Verification items for this drawing (mm, ordinates from the low corner). A direction names the side the tool comes from. Coordinates: 2 decimals unless noted, no trailing zeros. Order: outer loops, then holes, each group sorted by start corner. A loop starts at its lowest first (then second) coordinate and runs counter-clockwise, first axis right, second up. Notation, with made-up numbers: M 19.5,-7.5 L 78.5,-7.5 A23 ccw 78.5,1.5 Z; hole C 21,-35 d8. An arc over 180 degrees is marked long. Use CSV: the item, a comma, the result in double quotes. Start each with the question number.
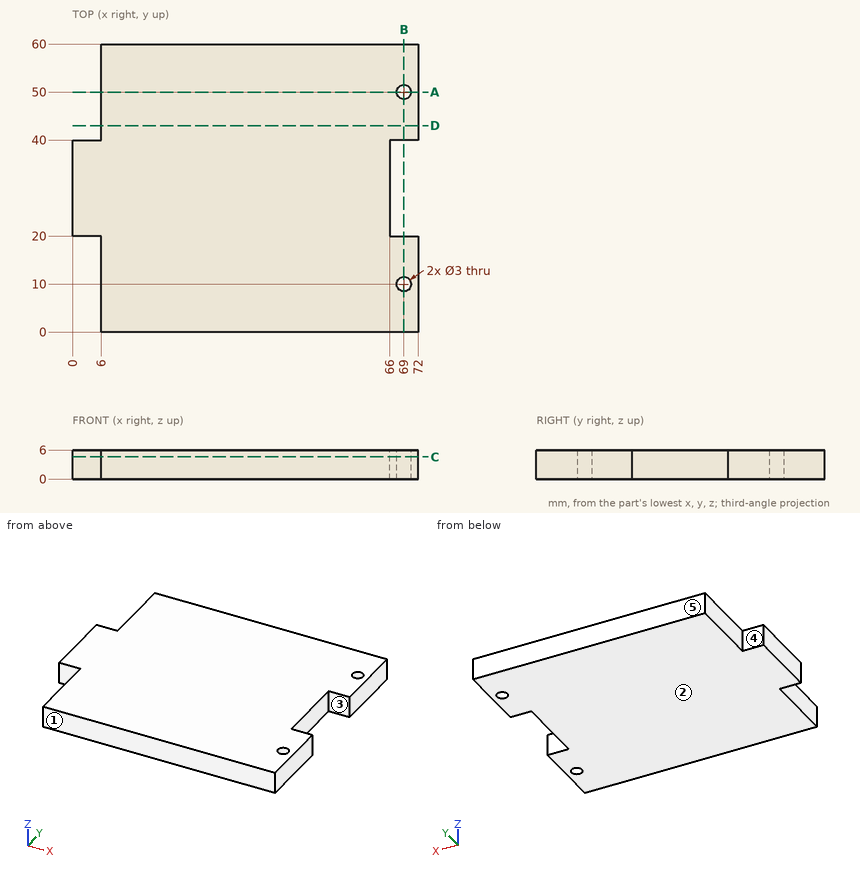
1) Section check D-D on y = 43. Record the boundary of the cut face in (x, z), then the cut area to 3 significant figures.
2) Draft check along Y on the marked faces 1, 2 and 3. Enter one of: +Y half, -Y half, draft (parallel to the pull), parting line (faces both ways), or undercut.
3) Section check A-A on y = 50. Record the boundary of the cut face in (x, z), then the cut area to 3 significant figures.
4) Set-up check for the marked faces 4 and 5: record each of +Z, -Z, +X, -X, +Y, -Y from which the full face is reachable in a straight line by a thin tool's end or side.
5) Gauge pin test, flat ends, axial feed: P1, Ø1.8, axis at y = 25.5, z = 2.5, coming from the +X side; P2, Ø3, axis at y = 50.5, z = 4, coming from the -X side; P3, Ø3, axis at x = 3.5, z = 4.5, coming from the -Y side. Record the tip position at first contact, or that the pin passes through.
6) Section check C-C on z = 4.6. Record the boundary of the cut face in (x, y), then the cut area to 3 significant figures.
7) Material ranges on line 1 along Y through (x, z) = (69, 2.15); line 2 along X through (y, z) = (50, 3); line 3 along X through (y, z) = (39, 2.7), recorded low to high.
8) Section check B-B on x = 69. Record the boundary of the cut face in (y, z).
Results are:
1,outline,"M 6,0 L 72,0 L 72,6 L 6,6 Z"
1,area,"396 mm²"
2,face 1,"-Y half"
2,face 2,"draft"
2,face 3,"undercut"
3,outline,"M 6,0 L 67.5,0 L 67.5,6 L 6,6 Z; M 70.5,0 L 72,0 L 72,6 L 70.5,6 Z"
3,area,"378 mm²"
4,face 4,"+Z, -Z, -X, +Y"
4,face 5,"+Z, -Z, +X, -X, +Y"
5,P1,"stops at x = 66"
5,P2,"stops at x = 6"
5,P3,"stops at y = 20"
6,outline,"M 0,20 L 6,20 L 6,0 L 72,0 L 72,20 L 66,20 L 66,40 L 72,40 L 72,60 L 6,60 L 6,40 L 0,40 Z; hole C 69,10 d3; hole C 69,50 d3"
6,area,"3,950 mm²"
7,line 1,"y = 0 to 8.5, 11.5 to 20, 40 to 48.5, 51.5 to 60"
7,line 2,"x = 6 to 67.5, 70.5 to 72"
7,line 3,"x = 0 to 66"
8,outline,"M 0,0 L 8.5,0 L 8.5,6 L 0,6 Z; M 11.5,0 L 20,0 L 20,6 L 11.5,6 Z; M 40,0 L 48.5,0 L 48.5,6 L 40,6 Z; M 51.5,0 L 60,0 L 60,6 L 51.5,6 Z"
